Verification items for this drawing (mm, ordinates from the low corner). A direction names the side the tool comes from. Give positions to 0.01 mm unless a question says otherwise; leave off trailing zeros. Loops run counter-clockwise (first coordinate to the right, second up) from the corner with the lowest first, then second, coordinate; pieces in that order, holes last. Notation, with made-up numbers: (64, -39.5) -> (103, -39.5) arc R11 ccw to (103, -22.5) -> close; hole circle Ø7 at (73.5, -32.5). An arc over 180 degrees is marked (long way). Write each question's results on one line, items separated by ' | '. Start each with the question number.
1) Sectioned sample at C-C on y = 23. Record the cut outline in (x, z), then the cut area to 3 significant figures.
2) Sectioned sample at B-B on z = 63. Record the cut outline in (x, y), then the cut area to 3 significant figures.
3) Sectioned sample at D-D on y = 8. Record the cut outline in (x, z).
4) Scan lines: line 1 (X direction, y = 26.5, z = 42.5); line 2 (X direction, y = 31.5, z = 24.5). Record each from-to range of solid material in increasing order. Write a range as from..to.
5) Draft check along Z on the marked faces 3, 4 and 5. Enter one of: pulls with the +Z half, pulls with the -Z half, needs draft (parallel to the pull), parting line crosses it, or undercut.
6) Depth check by flat-ended pin: pin 1 (8 mm diameter, centred on x = 91.5, y = 33.5, fed in from -Z); pin 2 (1 mm diameter, centred on y = 31.5, z = 53.5, fed in from -X); pin 3 (6 mm diameter, centred on y = 4.5, z = 121, fed in from +X); pin 4 (10 mm diameter, centred on x = 55, z = 134.5, fed in from +Y). Enter the tip coordinate at first touch or a pass-through.
7) Sectioned sample at A-A on x = 78.5. Record the cut outline in (y, z).
8) Set-up check for the marked faces 1 and 2: record each of +Z, -Z, +X, -X, +Y, -Y from which the full face is reachable in a straight line by a thin tool's end or side.
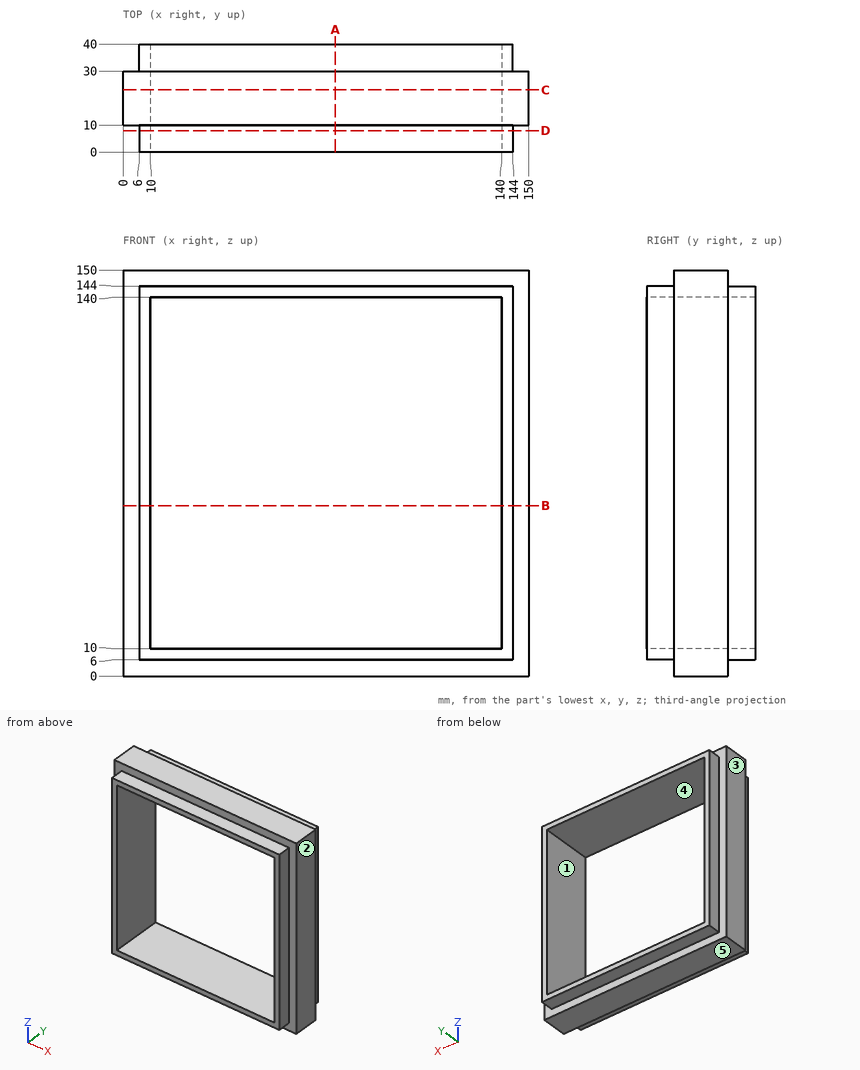
Result:
1) outline: (0, 0) -> (150, 0) -> (150, 150) -> (0, 150) -> close; hole (10, 10) -> (140, 10) -> (140, 140) -> (10, 140) -> close | area: 5,600 mm^2
2) outline: (0, 10) -> (6, 10) -> (6, 0) -> (10, 0) -> (10, 40) -> (6, 40) -> (6, 30) -> (0, 30) -> close; (140, 0) -> (144, 0) -> (144, 10) -> (150, 10) -> (150, 30) -> (144, 30) -> (144, 40) -> (140, 40) -> close | area: 560 mm^2
3) outline: (6, 6) -> (144, 6) -> (144, 144) -> (6, 144) -> close; hole (10, 10) -> (140, 10) -> (140, 140) -> (10, 140) -> close
4) line 1: 0..10, 140..150 | line 2: 6..10, 140..144
5) face 3: needs draft | face 4: undercut | face 5: pulls with the -Z half
6) pin 1: z = 0 | pin 2: x = 6 | pin 3: x = 144 | pin 4: through
7) outline: (0, 6) -> (10, 6) -> (10, 0) -> (30, 0) -> (30, 6) -> (40, 6) -> (40, 10) -> (0, 10) -> close; (0, 140) -> (40, 140) -> (40, 144) -> (30, 144) -> (30, 150) -> (10, 150) -> (10, 144) -> (0, 144) -> close
8) face 1: +Y, -Y | face 2: +Z, -Z, +X, +Y, -Y
